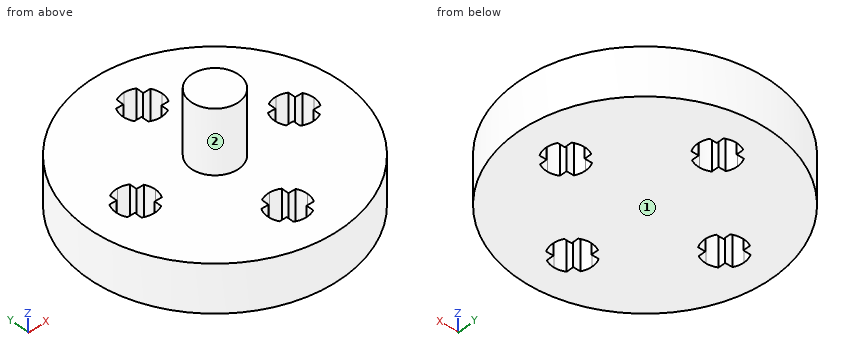
from build123d import *

# Parameters (mm, degrees)
CROQUIS1_R              = 16
SALIENTE_EXTRUIR1_DEPTH = 6
CROQUIS2_R              = 3
SALIENTE_EXTRUIR2_DEPTH = 8


with BuildPart() as part:
    # Croquis1 → Saliente-Extruir1 (new body)
    with BuildSketch(Plane.XY):
        Circle(CROQUIS1_R)
        with BuildLine():
            Line((2.165063509, 11.25), (1.25, 11.25))
            Line((1.25, 11.25), (1.25, 12.165063509))
            ThreePointArc((1.25, 12.165063509), (0.647047613, 12.414814566), (0, 12.5))
            ThreePointArc((0, 12.5), (-0.647047613, 12.414814566), (-1.25, 12.165063509))
            Line((-1.25, 12.165063509), (-1.25, 11.25))
            Line((-1.25, 11.25), (-2.165063509, 11.25))
            ThreePointArc((-2.165063509, 11.25), (-2.414814566, 10.647047613), (-2.5, 10))
            ThreePointArc((-2.5, 10), (-2.414814566, 9.352952387), (-2.165063509, 8.75))
            Line((-2.165063509, 8.75), (-1.25, 8.75))
            Line((-1.25, 8.75), (-1.25, 7.834936491))
            ThreePointArc((-1.25, 7.834936491), (-0.647047613, 7.585185434), (0, 7.5))
            ThreePointArc((0, 7.5), (0.647047613, 7.585185434), (1.25, 7.834936491))
            Line((1.25, 7.834936491), (1.25, 8.75))
            Line((1.25, 8.75), (2.165063509, 8.75))
            ThreePointArc((2.165063509, 8.75), (2.414814566, 9.352952387), (2.5, 10))
            ThreePointArc((2.5, 10), (2.414814566, 10.647047613), (2.165063509, 11.25))
        make_face(mode=Mode.SUBTRACT)
        with BuildLine():
            Line((11.25, -1.25), (12.165063509, -1.25))
            ThreePointArc((12.165063509, -1.25), (12.414814566, -0.647047613), (12.5, 0))
            ThreePointArc((12.5, 0), (12.414814566, 0.647047613), (12.165063509, 1.25))
            Line((12.165063509, 1.25), (11.25, 1.25))
            Line((11.25, 1.25), (11.25, 2.165063509))
            ThreePointArc((11.25, 2.165063509), (10.647047613, 2.414814566), (10, 2.5))
            ThreePointArc((10, 2.5), (9.352952387, 2.414814566), (8.75, 2.165063509))
            Line((8.75, 2.165063509), (8.75, 1.25))
            Line((8.75, 1.25), (7.834936491, 1.25))
            ThreePointArc((7.834936491, 1.25), (7.585185434, 0.647047613), (7.5, 0))
            ThreePointArc((7.5, 0), (7.585185434, -0.647047613), (7.834936491, -1.25))
            Line((7.834936491, -1.25), (8.75, -1.25))
            Line((8.75, -1.25), (8.75, -2.165063509))
            ThreePointArc((8.75, -2.165063509), (9.352952387, -2.414814566), (10, -2.5))
            ThreePointArc((10, -2.5), (10.647047613, -2.414814566), (11.25, -2.165063509))
            Line((11.25, -2.165063509), (11.25, -1.25))
        make_face(mode=Mode.SUBTRACT)
        with BuildLine():
            Line((-1.25, -11.25), (-1.25, -12.165063509))
            ThreePointArc((-1.25, -12.165063509), (-0.647047613, -12.414814566), (0, -12.5))
            ThreePointArc((0, -12.5), (0.647047613, -12.414814566), (1.25, -12.165063509))
            Line((1.25, -12.165063509), (1.25, -11.25))
            Line((1.25, -11.25), (2.165063509, -11.25))
            ThreePointArc((2.165063509, -11.25), (2.414814566, -10.647047613), (2.5, -10))
            ThreePointArc((2.5, -10), (2.414814566, -9.352952387), (2.165063509, -8.75))
            Line((2.165063509, -8.75), (1.25, -8.75))
            Line((1.25, -8.75), (1.25, -7.834936491))
            ThreePointArc((1.25, -7.834936491), (0.647047613, -7.585185434), (0, -7.5))
            ThreePointArc((0, -7.5), (-0.647047613, -7.585185434), (-1.25, -7.834936491))
            Line((-1.25, -7.834936491), (-1.25, -8.75))
            Line((-1.25, -8.75), (-2.165063509, -8.75))
            ThreePointArc((-2.165063509, -8.75), (-2.414814566, -9.352952387), (-2.5, -10))
            ThreePointArc((-2.5, -10), (-2.414814566, -10.647047613), (-2.165063509, -11.25))
            Line((-2.165063509, -11.25), (-1.25, -11.25))
        make_face(mode=Mode.SUBTRACT)
        with BuildLine():
            Line((-11.25, 1.25), (-12.165063509, 1.25))
            ThreePointArc((-12.165063509, 1.25), (-12.414814566, 0.647047613), (-12.5, 0))
            ThreePointArc((-12.5, 0), (-12.414814566, -0.647047613), (-12.165063509, -1.25))
            Line((-12.165063509, -1.25), (-11.25, -1.25))
            Line((-11.25, -1.25), (-11.25, -2.165063509))
            ThreePointArc((-11.25, -2.165063509), (-10.647047613, -2.414814566), (-10, -2.5))
            ThreePointArc((-10, -2.5), (-9.352952387, -2.414814566), (-8.75, -2.165063509))
            Line((-8.75, -2.165063509), (-8.75, -1.25))
            Line((-8.75, -1.25), (-7.834936491, -1.25))
            ThreePointArc((-7.834936491, -1.25), (-7.585185434, -0.647047613), (-7.5, 0))
            ThreePointArc((-7.5, 0), (-7.585185434, 0.647047613), (-7.834936491, 1.25))
            Line((-7.834936491, 1.25), (-8.75, 1.25))
            Line((-8.75, 1.25), (-8.75, 2.165063509))
            ThreePointArc((-8.75, 2.165063509), (-9.352952387, 2.414814566), (-10, 2.5))
            ThreePointArc((-10, 2.5), (-10.647047613, 2.414814566), (-11.25, 2.165063509))
            Line((-11.25, 2.165063509), (-11.25, 1.25))
        make_face(mode=Mode.SUBTRACT)
    extrude(amount=SALIENTE_EXTRUIR1_DEPTH)

    # Croquis2 → Saliente-Extruir2 (add)
    with BuildSketch(Plane.XY.offset(6)):
        Circle(CROQUIS2_R)
    extrude(amount=SALIENTE_EXTRUIR2_DEPTH)


solid = part.part
Work out the finished part from the listing and answer in its coordinate system (mm). Face numbers are marked on the shaded views. A direction names the side the tool comes from. Give positions to 0.01 mm unless a question says otherwise; leave off trailing zeros. Write each loop counter-clockwise with the first axis right and the second up, starting at its lowest first coordinate (ties: lowest second). Pieces come first, ordered by that corner, then holes. Notation, with made-up numbers: (-0.5, -10) - (14.5, -10) arc R13 cw to (14.5, -5) - close; hole circle Ø8 at (-20.75, -14). An arc over 180 degrees is marked (long way). One line per item, written item: value. Start each with the question number.
1. For the marked faces 1 and 2, determine the directions among +Z, -Z, +X, -X, +Y, -Y from which every point of the face is accessible in a straight line to the end or side of a thin tool.
2. Find section D-D (x = 14.5). Write down the section's boundary in (y, z), then the cut area to 3 significant figures.
3. Find section C-C (z = 11). Write down the section's boundary in (x, y), then the cut area to 3 significant figures.
4. Given pin 1 (0.5 mm diameter, centred on y = 11.5, z = 4, fed in from +X); pin 2 (0.5 mm diameter, centred on x = -1.5, z = 3, fed in from -Y); pin 3 (0.7 mm diameter, centred on x = -8.5, z = 2, fed in from -Y); pin 4 (6 mm diameter, centred on x = 2.5, z = 5.5, fed in from +Y), each flat-ended and moving along its own axis, determine where each tip first touches the part or whether it passes through.
5. Find section A-A (y = 0.5). Write down the section's boundary in (x, z), then the cut area to 3 significant figures.
6. Consider probe 1 along Y at (x, z) = (-0.5, 3); probe 2 along Z at (x, y) = (-3, 14); probe 3 along Y at (x, z) = (-12, 2). Determine where each line is inside the solid, lowest interval first.
7. Find section B-B (z = 3). State how many separate pieces and enclosed holes the cut face has, then the cut area to 3 significant figures.
Geometry results:
1. face 1: -Z, +X, -X, +Y, -Y
1. face 2: +Z
2. outline: (-6.76, 0) - (6.76, 0) - (6.76, 6) - (-6.76, 6) - close
2. area: 81.2 mm2
3. outline: circle Ø6 at (0, 0)
3. area: 28.3 mm2
4. pin 1: x = 11.38
4. pin 2: y = -15.95
4. pin 3: y = -13.77
4. pin 4: y = 16
5. outline: (-15.99, 0) - (-12.45, 0) - (-12.45, 6) - (-15.99, 6) - close; (-7.55, 0) - (7.55, 0) - (7.55, 6) - (2.96, 6) - (2.96, 14) - (-2.96, 14) - (-2.96, 6) - (-7.55, 6) - close; (12.45, 0) - (15.99, 0) - (15.99, 6) - (12.45, 6) - close
5. area: 180 mm2
6. probe 1: -15.99 to -12.45, -7.55 to 7.55, 12.45 to 15.99
6. probe 2: 0 to 6
6. probe 3: -10.58 to -1.25, 1.25 to 10.58
7. separate pieces: 1
7. enclosed holes: 4
7. area: 734 mm2
